Here's how the part is built. I have some questions about the finished solid (model axes, mm). A direction names the side the tool comes from. Coordinates: 2 decimals unless noted, no trailing zeros. Write each loop counter-clockwise with the first axis right and the second up, starting at its lowest first coordinate (ties: lowest second). Pieces come first, ordered by that corner, then holes.
Item 1: We'd pull the mould along Z, two halves only. Please class faces 3 (the face through (-11.5, 6.1, 0)), 4 (the face through (0, 0, 0)), 5 (the face through (-6, 1, 0)): +Z half, -Z half, draft (parallel to the pull), parting line (faces both ways), or undercut.
Item 2: If we section it at C-C (z = -5.5): Please give me the cut outline in (x, y).
Item 3: If we section it at D-D (x = 3): Please give me the cut outline in (y, z), then the cut area to 3 significant figures.
Item 4: For faces 1 (the face through (-3.555, 1.479, -2.726)), 2 (the face through (5.2, 0, 3.5)), which set-ups out of +Z, -Z, +X, -X, +Y, -Y let a thin tool reach every point of the face, with its end or its side?
Item 5: I'm going to push flat-ended pins straight in: pin 1 Ø3 at (x, y) = (-8, 4.5) entering from -Z; pin 2 Ø3 at (y, z) = (1.5, -6) entering from +X; pin 3 Ø1.5 at (x, y) = (6, 8.5) entering from +Z. Where does each tip first touch, or does it pass through?
Item 6: If I drill on line 1 (Z direction, x = 0, y = 2.25); line 2 (Z direction, x = -9.5, y = 2.5), over which ranges is the centre line in solid material (lowest first)?
Item 7: If we section it at B-B (x = 0): Please give me the cut outline in (y, z).
Item 8: If we section it at A-A (y = 8): Please give me the cut outline in (x, z).
Autodesk Inventor part; units mm, degrees
ref_plane "YZ Plane" through (0, 0, 0) normal (1, 0, 0) x (0, 1, 0)
ref_plane "XZ Plane" through (0, 0, 0) normal (0, 1, 0) x (-1, 0, 0)
ref_plane "XY Plane" through (0, 0, 0) normal (0, 0, 1) x (1, 0, 0)
sketch "Sketch1" plane through (0, 0, 0) normal (0, 1, 0) x (-1, 0, 0)
  circle A0 centre (0, 0) radius 9.5
  dimension "d0" = 19
extrude "Extrusion1" add sketch "Sketch1" along normal blind 12
sketch "Sketch3" plane through (0, 0, 0) normal (0, -1, 0) x (1, 0, 0)
  circle A0 centre (0, 0) radius 4.48
  circle A1 centre (0, 0) radius 6
  dimension "d5" = 12
  dimension "d6" = 1.52
extrude "Extrusion3" cut sketch "Sketch3" against normal blind 3
sketch "Sketch4" plane through (0, 12, 0) normal (0, 1, 0) x (1, 0, 0)
  circle A0 centre (0, 0) radius 9.5
  circle A1 centre (-9.5, 0) radius 2
  line L0 (-15.7, 0) -> (13.7, 0)
  point P0 (-9.2895, 1.9889)
  point P1 (-9.2895, -1.9889)
  dimension "d10" = 4
extrude "Extrusion4" add sketch "Sketch4" against normal up to surface (12 mm away) contours A0 L0 A1 | A1 L0 A0 picked at (-10.0838, 0.5297) picked at (-10.0838, -0.5297)
pattern_circular "Circular Pattern1" count 4 over 360 about axis through (0, 0, 0) along (0, 1, 0) of "Extrusion4"
properties part number "Soporte Resorte"
Answer list:
1. face 3: parting line
1. face 4: draft
1. face 5: undercut
2. outline: (-7.75, 0) - (-2.4, 0) - (-2.4, 3) - (2.4, 3) - (2.4, 0) - (7.75, 0) - (7.75, 12) - (-7.75, 12) - close
3. outline: (0, -9.01) - (12, -9.01) - (12, 9.01) - (0, 9.01) - (0, 5.2) - (3, 5.2) - (3, 3.33) - (0, 3.33) - (0, -3.33) - (3, -3.33) - (3, -5.2) - (0, -5.2) - close
3. area: 205 mm2
4. face 1: -Y
4. face 2: +Z, -Z, +X, -X, -Y
5. pin 1: stops at z = -6.93
5. pin 2: stops at x = 8.37
5. pin 3: stops at z = 7.92
6. line 1: z = -11.5 to -6, -4.48 to 4.48, 6 to 11.5
6. line 2: z = -2 to 2
7. outline: (0, -11.5) - (12, -11.5) - (12, 11.5) - (0, 11.5) - (0, 6) - (3, 6) - (3, 4.48) - (0, 4.48) - (0, -4.48) - (3, -4.48) - (3, -6) - (0, -6) - close
8. outline: (-9.29, -1.99) arc R9.5 ccw to (-1.99, -9.29) arc R2 ccw (long way) to (1.99, -9.29) arc R9.5 ccw to (9.29, -1.99) arc R2 ccw (long way) to (9.29, 1.99) arc R9.5 ccw to (1.99, 9.29) arc R2 ccw (long way) to (-1.99, 9.29) arc R9.5 ccw to (-9.29, 1.99) arc R2 ccw (long way) to start
